Read the model definition and answer for the solid it produces. Units are mm, in the model's axes. A direction names the side the tool comes from. Coordinates: 2 decimals unless noted, no trailing zeros. Write each loop counter-clockwise with the first axis right and the second up, starting at its lowest first coordinate (ties: lowest second). Pieces come first, ordered by that corner, then holes. Notation, with made-up numbers: (-26.5, 25) -> (-10.5, 25) arc R10 cw to (-10.5, 31) -> close; hole circle Ø6 at (35, 77.25). An arc over 180 degrees is marked (long way). Answer in a Markdown table with one row per item. Add a question column.
Item 1: Given pin 1 Ø12.5 at (x, z) = (-4, 11.5) entering from +Y, flat-ended and moving along its own axis, determine where the tip first touches the part or whether it passes through.
Item 2: Straight lines are drawn through the part: line 1 (Z direction, x = 0, y = -6.25); line 2 (Z direction, x = 0, y = -1.2); line 3 (X direction, y = -1, z = 12). For each, find the intervals that lie inside material, in ascending order. Write a range as from..to.
Item 3: For a pull along X with two mould halves and no side action, classify faces 1 (the face through (5, -1.588, 12)), 2 (the face through (-3, -9.525, 0)), 3 (the face through (185.738, -5, 0)) as +X half, -X half, draft (parallel to the pull), parting line (faces both ways), or undercut.
Item 4: Section A-A on x = 0 is taken. Write down the section's boundary in (y, z) (1 decimal), then the cut area to 3 significant figures.
Item 5: Which of the six approach directions +Z, -Z, +X, -X, +Y, -Y give full straight-line access (tool end or side, diameter ignored) to faces 4 (the face through (-2.753, -0.783, -0.492)), 5 (the face through (-1.032, -5.501, 7.257))?
```python
from build123d import *

# Parameters (mm, degrees)
F0_W     = 371.475
F0_H     = 55.5625
F0_R     = 12.7
F0_R_2   = 4.7625
F1_DEPTH = 9.525
F2_DEPTH = 1.5875


with BuildPart() as f1:
    # F0 (on Front) → F1 (new body)
    with BuildSketch(Plane.XZ):
        Rectangle(F0_W, F0_H)
        with Locations((0, 11.90625)):
            Circle(F0_R, mode=Mode.SUBTRACT)
        with Locations((0, 11.90625)):
            Circle(F0_R)
        with Locations((0, 11.90625)):
            Circle(F0_R_2, mode=Mode.SUBTRACT)
    extrude(amount=F1_DEPTH)

    # F0 (on Front) → F2 (cut)
    with BuildSketch(Plane.XZ):
        with Locations((0, 11.90625)):
            Circle(F0_R)
        with Locations((0, 11.90625)):
            Circle(F0_R_2, mode=Mode.SUBTRACT)
    extrude(amount=F2_DEPTH, mode=Mode.SUBTRACT)


solid = f1.part
```
Results below:
| question | item | result |
|---|---|---|
| 1 | pin 1 | stops at y = -1.59 |
| 2 | line 1 | z = -27.78..7.14, 16.67..27.78 |
| 2 | line 2 | z = -27.78..-0.79, 24.61..27.78 |
| 2 | line 3 | x = -185.74..-12.7, 12.7..185.74 |
| 3 | face 1 | undercut |
| 3 | face 2 | draft |
| 3 | face 3 | +X half |
| 4 | outline | (-9.5, -27.8) -> (0, -27.8) -> (0, -0.8) -> (-1.6, -0.8) -> (-1.6, 7.1) -> (-9.5, 7.1) -> close; (-9.5, 16.7) -> (-1.6, 16.7) -> (-1.6, 24.6) -> (0, 24.6) -> (0, 27.8) -> (-9.5, 27.8) -> close |
| 4 | area | 413 mm2 |
| 5 | face 4 | +Y |
| 5 | face 5 | +Y, -Y |
